Part model, mm, in its own coordinate system. A direction names the side the tool comes from. Round coordinates to 2 decimals unless told otherwise and drop trailing zeros. Write each loop counter-clockwise with the first axis right and the second up, starting at its lowest first coordinate (ties: lowest second). Pieces come first, ordered by that corner, then holes. Notation, with made-up numbers: (57.25, -32) -> (87.25, -32) arc R31 ccw to (87.25, -8) -> close; hole circle Ø6 at (-34.5, 46.5). An arc over 180 degrees is marked (long way). Use CSV: the item, a comma, the result in double quotes. Start each with the question number.
(1) Saw through at B-B (z = 10.5). Give the cut face in (x, y), plus the area to 3 significant figures.
(2) Saw through at D-D (x = 22). Give the cut face in (y, z), plus the area to 3 significant figures.
(3) Which spindle directions (+Z, -Z, +X, -X, +Y, -Y) get a long thin tool onto all of the face, cutting with end or side? Do faces 5 (the flat face through (-20.5, 45, -0.1)), 6 (the flat face through (20, 25, 0)). Say none if no direction does.
(4) Drop a flat-ended pin along its axis: pin 1 (12 mm diameter, centred on x = 9, z = 8.5, fed in from +Y). Give the stop position or say it passes through.
(5) Probe line 1 (X direction, y = 29.5, z = 13.5); line 2 (Y direction, x = -4, z = -12). List the from-to ranges inside material, lowest first. Write a range as [from, to].
(6) Saw through at A-A (y = 32). Give the cut face in (x, z), plus the area to 3 significant figures.
(7) Two-plate mould, pull along Z, no slides. Class faces 1 (the flat face through (25, 27, 0)), 2 (the cylindrical face through (-22.291, 27.498, -22.143)), 3 (the cylindrical face through (0.217, 2.857, 22.291)), 4 (the flat face through (-20, 25, 0)): released by +Z, released by -Z, zero draft, split by the parting line, or undercut.
(8) Saw through at C-C (x = 13.5). Give the cut face in (y, z), plus the area to 3 significant figures.
```python
from build123d import *

# Parameters (mm, degrees)
SKETCH1_W           = 50
SKETCH1_H           = 50
BOSS_EXTRUDE1_DEPTH = 45
SHELL1_T            = -5
FILLET1_R           = 4.5
FILLET2_R           = 9.5


with BuildPart() as part:
    # Sketch1 → Boss-Extrude1 (new body)
    with BuildSketch(Plane(origin=(0, 0, 0), x_dir=(1, 0, 0), z_dir=(0, 1, 0))):
        Rectangle(SKETCH1_W, SKETCH1_H)
    extrude(amount=BOSS_EXTRUDE1_DEPTH)

    # Shell1
    shell1_openings = [part.faces().sort_by_distance(p)[0] for p in [
        (0, 45, 0),
    ]]
    offset(amount=SHELL1_T, openings=shell1_openings, kind=Kind.INTERSECTION)

    # Fillet1
    fillet1_edges = [part.edges().sort_by_distance(p)[0] for p in [
        (20, 25, 20),
        (20, 25, -20),
        (-20, 25, -20),
        (-20, 25, 20),
    ]]
    fillet(fillet1_edges, radius=FILLET1_R)

    # Fillet2
    fillet2_edges = [part.edges().sort_by_distance(p)[0] for p in [
        (0, 0, 25),
        (-25, 0, 0),
        (0, 0, -25),
        (25, 0, 0),
        (25, 22.5, 25),
        (-25, 22.5, 25),
        (-25, 22.5, -25),
        (25, 22.5, -25),
    ]]
    fillet(fillet2_edges, radius=FILLET2_R)


solid = part.part
```
Answers:
1,outline,"(-25, 9.5) arc R9.5 ccw to (-15.5, 0) -> (15.5, 0) arc R9.5 ccw to (25, 9.5) -> (25, 45) -> (20, 45) -> (20, 5) -> (-20, 5) -> (-20, 45) -> (-25, 45) -> close"
1,area,"611 mm²"
2,outline,"(2.57, -15.5) arc R6.93 ccw to (9.5, -22.43) -> (45, -22.43) -> (45, 22.43) -> (9.5, 22.43) arc R6.93 ccw to (2.57, 15.5) -> close"
2,area,"1,880 mm²"
3,face 5,"+Z, -Z, +X, -X, +Y"
3,face 6,"+Y"
4,pin 1,"stops at y = 5"
5,line 1,"x = [-25, -20], [20, 25]"
5,line 2,"y = [0, 5]"
6,outline,"(-25, -15.5) arc R9.5 ccw to (-15.5, -25) -> (15.5, -25) arc R9.5 ccw to (25, -15.5) -> (25, 15.5) arc R9.5 ccw to (15.5, 25) -> (-15.5, 25) arc R9.5 ccw to (-25, 15.5) -> close; hole (-20, -15.5) arc R4.5 ccw to (-15.5, -20) -> (15.5, -20) arc R4.5 ccw to (20, -15.5) -> (20, 15.5) arc R4.5 ccw to (15.5, 20) -> (-15.5, 20) arc R4.5 ccw to (-20, 15.5) -> close"
6,area,"840 mm²"
7,face 1,"zero draft"
7,face 2,"released by -Z"
7,face 3,"released by +Z"
7,face 4,"undercut"
8,outline,"(0, -15.5) arc R9.5 ccw to (9.5, -25) -> (45, -25) -> (45, -20) -> (5, -20) -> (5, 20) -> (45, 20) -> (45, 25) -> (9.5, 25) arc R9.5 ccw to (0, 15.5) -> close"
8,area,"611 mm²"
